Can you work these out from the model? Positions are in its coordinate system, mm. Face numbers are marked on the shaded views. A direction names the side the tool comes from. Round coordinates to 2 decimals unless told otherwise and drop trailing zeros. Loops run counter-clockwise (first coordinate to the right, second up) from the corner with the lowest first, then second, coordinate; pieces in that order, holes last. Notation, with made-up numbers: M 9,-4.5 L 22,-4.5 A30 cw 22,29.5 Z; hole C 7.25,26.25 d10. An arc over 180 degrees is marked long. Answer as CSV lines item,"result".
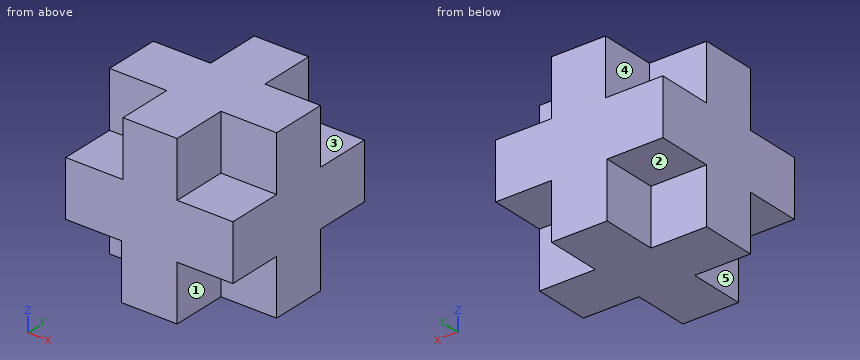
from build123d import *

# Parameters (mm, degrees)
F0_W     = 60
F0_H     = 60
F1_DEPTH = 60
F2_W     = 20.549892
F2_H     = 20
F2_W_2   = 20
F3_DEPTH = 20
F4_W     = 20
F4_H     = 20
F5_DEPTH = 20


with BuildPart() as f1:
    # F0 (on Top) → F1 (new body)
    with BuildSketch(Plane.XY):
        Rectangle(F0_W, F0_H)
    extrude(amount=F1_DEPTH)

    # F2 (on face) → F3 (cut)
    with BuildSketch(Plane.XY.offset(60)):
        with Locations((-19.725054, 20)):
            Rectangle(F2_W, F2_H)
        with Locations((20, 20)):
            Rectangle(F2_W_2, F2_H)
        with Locations((20, -20)):
            Rectangle(F2_W_2, F2_H)
        with Locations((-19.725054, -20)):
            Rectangle(F2_W, F2_H)
    extrude(amount=-F3_DEPTH, mode=Mode.SUBTRACT)

    # F4 (on face) → F5 (cut)
    with BuildSketch(Plane(origin=(0, 0, 0), x_dir=(1, 0, 0), z_dir=(0, 0, -1))):
        with Locations((20, -20)):
            Rectangle(F4_W, F4_H)
        with Locations((-20, -20)):
            Rectangle(F4_W, F4_H)
        with Locations((-20, 20)):
            Rectangle(F4_W, F4_H)
        with Locations((20, 20)):
            Rectangle(F4_W, F4_H)
    extrude(amount=-F5_DEPTH, mode=Mode.SUBTRACT)


solid = f1.part
Item 1: Will these pins go through, and if not, where does the flat tip stop? pin 1 (10 mm diameter, centred on y = -17, z = 6.5, fed in from +X); pin 2 (10 mm diameter, centred on x = 20, z = 7, fed in from +Y); pin 3 (22 mm diameter, centred on x = 24.5, z = 7, fed in from -Y).
Output:
pin 1,"stops at x = 10"
pin 2,"stops at y = 10"
pin 3,"stops at y = -10"
Item 2: On a 3-axis mill with a long thin cutter (end or side, diameter ignored), from which of +Z, -Z, +X, -X, +Y, -Y can I reach the whole of each face in a straight line? I mean the marked faces 1, 2, 3, 4 and 5. Say none if no direction works.
Output:
face 1,"-Z, +X, -Y"
face 2,"-Z, -X, +Y"
face 3,"+Z, +X, +Y"
face 4,"+Z, -X, +Y"
face 5,"-Z, -X, -Y"
Item 3: If we section it at B-B on y = -24: Write out the boundary of the cut face in (x, z).
Output:
outline,"M -30,20 L -10,20 L -10,0 L 10,0 L 10,20 L 30,20 L 30,40 L 10,40 L 10,60 L -9.45,60 L -9.45,40 L -30,40 Z"
Item 4: If I drill on line 1 along X through (y, z) = (-18.5, 41); line 2 along X through (y, z) = (19.5, 19), over which ranges is the centre line in solid material (lowest first)? Write a range as from..to.
Output:
line 1,"x = -9.45..10"
line 2,"x = -10..10"
Item 5: If we section it at A-A on z = 19: Write out the boundary of the cut face in (x, y).
Output:
outline,"M -30,-10 L -10,-10 L -10,-30 L 10,-30 L 10,-10 L 30,-10 L 30,10 L 10,10 L 10,30 L -10,30 L -10,10 L -30,10 Z"
